The listing builds one solid part. Answer for the finished solid, in the listing's coordinates (mm). A direction names the side the tool comes from. Give positions to 0.01 mm unless a question says otherwise; leave off trailing zeros. Order: outer loops, then holes, each group sorted by start corner. A loop starts at its lowest first (then second) coordinate and runs counter-clockwise, first axis right, second up. Notation, with made-up numbers: (30.5, 68.5) - (71.5, 68.5) arc R12 ccw to (71.5, 73.5) - close; hole circle Ø11 at (37.25, 11.25). An arc over 180 degrees is marked (long way). Answer in a Markdown table with one row per item.
from build123d import *

# Parameters (mm, degrees)
BOSS_EXTRUDE1_DEPTH = 120
BOSS_EXTRUDE2_DEPTH = 30
FILLET1_R           = 10
FILLET2_R           = 10
CUT_EXTRUDE1_DEPTH  = 85


with BuildPart() as part:
    # Sketch1 → Boss-Extrude1 (new body)
    with BuildSketch(Plane.XY):
        Polygon((0, 0), (15.9, 0), (15.9, 11.8), (-15.9, 11.8), (-15.9, 0), align=None)
    extrude(amount=-BOSS_EXTRUDE1_DEPTH)

    # Sketch2 → Boss-Extrude2 (add)
    with BuildSketch(Plane.XY.offset(-5)):
        with BuildLine():
            Line((-15.9, 15.45), (17.7, 15.45))
            ThreePointArc((17.7, 15.45), (23.003300859, 13.253300859), (25.2, 7.95))
            Line((25.2, 7.95), (25.2, -4.05))
            Line((25.2, -4.05), (25.2, -6.799114346))
            ThreePointArc((25.2, -6.799114346), (24.015595093, -9.187338468), (21.397590361, -9.689813011))
            ThreePointArc((21.397590361, -9.689813011), (0, -6.775110745), (-21.397590361, -9.689813011))
            ThreePointArc((-21.397590361, -9.689813011), (-24.015595093, -9.187338468), (-25.2, -6.799114346))
            Line((-25.2, -6.799114346), (-25.2, -4.05))
            Line((-25.2, -4.05), (-25.2, 7.95))
            ThreePointArc((-25.2, 7.95), (-23.003300859, 13.253300859), (-17.7, 15.45))
            Line((-17.7, 15.45), (-15.9, 15.45))
        make_face()
    extrude(amount=-BOSS_EXTRUDE2_DEPTH)

    # Fillet1
    # the kernel refuses this fillet: 10 mm, written as the material it takes off along each edge
    with BuildSketch(Plane(origin=(15.9, -21.650635095, 0), x_dir=(0, 0, -1), z_dir=(0, 1, 0))) as fillet1_piece_1:
        with BuildLine():
            CenterArc((10, 8.660254038), FILLET1_R, 180, 60)
            Line((0, 8.660254038), (-0.2, 8.660254038))
            Line((-0.2, 8.660254038), (-0.2, 0))
            Line((-0.2, 0), (0, -0.2))
            ThreePointArc((0, -0.2), (2.5, -0.2), (4.9, -0.173205081))
            Line((4.9, -0.173205081), (5, 0))
        make_face()
    extrude(amount=55.101270189, mode=Mode.SUBTRACT)

    # Fillet2
    # the kernel refuses this fillet: 10 mm, written as the material it takes off along each edge
    with BuildSketch(Plane(origin=(-15.9, 33.450635095, 0), x_dir=(1, 0, 0), z_dir=(0, -1, 0))) as fillet2_piece_1:
        with BuildLine():
            CenterArc((8.660254038, -10), FILLET2_R, 90, 60)
            Line((0, -5), (-0.173205081, -4.9))
            ThreePointArc((-0.173205081, -4.9), (-0.2, -2.5), (-0.2, 0))
            Line((-0.2, 0), (0, 0.2))
            Line((0, 0.2), (8.660254038, 0.2))
            Line((8.660254038, 0.2), (8.660254038, 0))
        make_face()
    extrude(amount=55.101270189, mode=Mode.SUBTRACT)

    # Sketch3 → Cut-Extrude1 (cut)
    with BuildSketch(Plane(origin=(25.2, 0, 0), x_dir=(0, 0, -1), z_dir=(1, 0, 0))):
        Polygon((20, -4.799114346), (30, -4.799114346), (30, -0.799114346), (10, -0.799114346), (10, -4.799114346), align=None)
    extrude(amount=-CUT_EXTRUDE1_DEPTH, mode=Mode.SUBTRACT)


solid = part.part
Item 1: Find section B-B on y = -3.25. Write down the section's boundary in (x, z), then the cut area to 3 significant figures.
Answer block:
| item | result |
|---|---|
| outline | (-25.2, -35) - (25.2, -35) - (25.2, -30) - (-25.2, -30) - close; (-25.2, -10) - (25.2, -10) - (25.2, -5) - (-25.2, -5) - close |
| area | 504 mm² |
Item 2: Which of the six approach directions +Z, -Z, +X, -X, +Y, -Y give full straight-line access (tool end or side, diameter ignored) to faces 1 (the face through (0, -3, -10)), 2 (the face through (0, 11.8, -2)), 3 (the face through (0, 0, -77)), 4 (the face through (25.2, 2, -20)), 5 (the face through (-15.9, 6, -77))?
Answer block:
| item | result |
|---|---|
| face 1 | +X, -X |
| face 2 | +Z, +X, -X, +Y |
| face 3 | -Z, +X, -X, -Y |
| face 4 | +Z, -Z, +X, +Y, -Y |
| face 5 | -Z, -X, +Y, -Y |
Item 3: Consider line 1 (Z direction, x = 1.5, y = -4.25); line 2 (Y direction, x = -1, z = -91.5); line 3 (Z direction, x = -10, y = -5.5). Determine where each line is inside the solid, lowest interval first.
Answer block:
| item | result |
|---|---|
| line 1 | -35 to -30, -10 to -5 |
| line 2 | 0 to 11.8 |
| line 3 | -35 to -5 |
Item 4: Find section C-C on x = 5.5. Write down the section's boundary in (y, z).
Answer block:
| item | result |
|---|---|
| outline | (-6.96, -35) - (0, -35) - (0, -120) - (11.8, -120) - (11.8, -35) - (15.45, -35) - (15.45, -5) - (11.8, -5) - (11.8, 0) - (0, 0) - (0, -5) - (-6.96, -5) - close; hole (-4.8, -30) - (-0.8, -30) - (-0.8, -10) - (-4.8, -10) - close |
Item 5: Find section D-D on y = 5.25. Write down the section's boundary in (x, z), then the cut area to 3 significant figures.
Answer block:
| item | result |
|---|---|
| outline | (-25.2, -35) - (-15.9, -35) - (-15.9, -120) - (15.9, -120) - (15.9, -35) - (25.2, -35) - (25.2, -5) - (15.9, -5) arc R10 ccw to (7.24, 0) - (-7.24, 0) arc R10 ccw to (-15.9, -5) - (-25.2, -5) - close |
| area | 4,350 mm² |
Item 6: Find section A-A on z = -12. Write down the section's boundary in (x, y), then the cut area to 3 significant figures.
Answer block:
| item | result |
|---|---|
| outline | (-25.2, -6.8) arc R3 ccw to (-21.4, -9.69) arc R80 cw to (21.4, -9.69) arc R3 ccw to (25.2, -6.8) - (25.2, -4.8) - (-25.2, -4.8) - close; (-25.2, -0.8) - (25.2, -0.8) - (25.2, 7.95) arc R7.5 ccw to (17.7, 15.45) - (-17.7, 15.45) arc R7.5 ccw to (-25.2, 7.95) - close |
| area | 955 mm² |
Item 7: Each of these flat-tipped pins is pushed along its axis until it touches: P1, Ø4, axis at x = -3.5, z = -3.5, coming from the -Y side; P2, Ø5, axis at x = -14.5, z = -18.5, coming from the -Y side; P3, Ø2, axis at x = -8.5, z = -80.5, coming from the -Y side; P4, Ø3, axis at x = -18.5, z = -42, coming from the -Y side. Where does it stop, or does it pass through?
Answer block:
| item | result |
|---|---|
| P1 | y = -6.92 |
| P2 | y = -8.6 |
| P3 | y = 0 |
| P4 | through |
Item 8: Determine the mould class of faces 6 (the face through (15.9, 6, -77)), 7 (the face through (-23.061, 13.195, -19.79)), 8 (the face through (0, -0.799, -20)) for opening direction Y: pulls with the +Y half, pulls with the -Y half, needs draft (parallel to the pull), parting line crosses it, or undercut.
Answer block:
| item | result |
|---|---|
| face 6 | needs draft |
| face 7 | pulls with the +Y half |
| face 8 | undercut |
